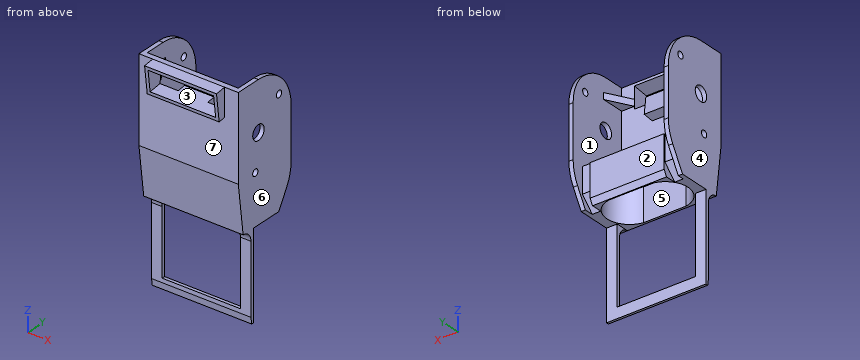
from build123d import *

# Parameters (mm, degrees)
EXTRUDE_1_DEPTH          = 15.5
SKETCH_2_W               = 41
SKETCH_2_H               = 24
EXTRUDE_2_DEPTH          = 2.5
EXTRUDE_3_DEPTH          = 41
EXTRUDE_5_DEPTH          = 1
EXTRUDE_6_DEPTH          = 1
EXTRUDE_7_DEPTH          = 2
CUT_EXTRUDE_1_REACH      = 81.452
SKETCH_10_R              = 1.6
SKETCH_10_R_2            = 3.5
EXTRUDE_8_DEPTH          = 2
CUT_EXTRUDE_2_REACH      = 82.601
SKETCH_12_R              = 3.5
SKETCH_12_R_2            = 1.6
EXTRUDE_9_DEPTH          = 43
EXTRUDE_10_DEPTH         = 3
EXTRUDE_11_DEPTH         = 1.5
FILLET_1_R               = 5
SKETCH_21_W              = 35
SKETCH_21_H              = 18
EXTRUDE_12_DEPTH         = 0.5
CHAMFER_1_SIZE           = 6
CUT_EXTRUDE_4_DEPTH      = 10
CUT_EXTRUDE_4_DEPTH_BACK = 0.7
SKETCH_24_W              = 99.76929375
SKETCH_24_H              = 144.1272379
CHAMFER_2_SIZE           = 15
CHAMFER_2_SIZE2          = 8.660254038
CHAMFER_3_SIZE           = 7.5
CHAMFER_3_SIZE2          = 12.990381057
CHAMFER_4_SIZE           = 1.5
CHAMFER_4_SIZE2          = 2.598076211
EXTRUDE_13_REACH         = 76.53
SKETCH_25_W              = 34
SKETCH_25_H              = 13
CUT_EXTRUDE_5_REACH      = 76.53
SKETCH_26_W              = 31
SKETCH_26_H              = 10
EXTRUDE_14_REACH         = 72.111
SKETCH_27_W              = 14
SKETCH_27_H              = 8
FILLET_2_R               = 20
FILLET_3_R               = 20


with BuildPart() as part:
    # ｽｹｯﾁ1 → ﾎﾞｽ - 押し出し1 (new body)
    with BuildSketch(Plane.XY):
        Polygon((10.055611053, 12.166632755), (-10.143634653, 12.166632755), (-20.595217471, 12.166632755), (-20.595217471, -0.083367245), (-20.595217471, -11.833367245), (-10.143634653, -11.833367245), (10.055611053, -11.833367245), (20.404782529, -11.833367245), (20.404782529, 0.125988678), (20.404782529, 12.166632755), align=None)
        with BuildLine():
            Line((9.95247038, 10.766632755), (-10.04752962, 10.766632755))
            ThreePointArc((-10.04752962, 10.766632755), (-19.245217471, 0.166632755), (-10.04752962, -10.433367245))
            Line((-10.04752962, -10.433367245), (9.95247038, -10.433367245))
            ThreePointArc((9.95247038, -10.433367245), (19.054782529, 0.166632755), (9.95247038, 10.766632755))
        make_face(mode=Mode.SUBTRACT)
    extrude(amount=EXTRUDE_1_DEPTH)

    # ｽｹｯﾁ2 → ﾎﾞｽ - 押し出し2 (add)
    with BuildSketch(Plane.XY.offset(15.5)):
        with Locations((-0.095217471, 0.166632755)):
            Rectangle(SKETCH_2_W, SKETCH_2_H)
    extrude(amount=EXTRUDE_2_DEPTH)

    # ｽｹｯﾁ3 → ﾎﾞｽ - 押し出し3 (add)
    with BuildSketch(Plane.ZY.offset(20.595217471)):
        Polygon((0, -12.15110343), (17.677739562, -14.384321281), (18, -11.833367245), (0, -11.833367245), align=None)
    extrude(amount=-EXTRUDE_3_DEPTH)

    # ｽｹｯﾁ5 → ﾎﾞｽ - 押し出し5 (add)
    with BuildSketch(Plane.ZY.offset(20.595217471)):
        Polygon((0, 12.166632755), (0, -12.15110343), (17.677739562, -14.384321281), (18, -11.833367245), (18, 12.166632755), align=None)
    extrude(amount=EXTRUDE_5_DEPTH)

    # ｽｹｯﾁ7 → ﾎﾞｽ - 押し出し6 (add)
    with BuildSketch(Plane(origin=(20.404782529, 0, 0), x_dir=(0, 0, -1), z_dir=(1, 0, 0))):
        Polygon((0, -12.15110343), (0, 12.166632755), (-18, 12.166632755), (-18, -11.833367245), (-17.677739562, -14.384321281), align=None)
    extrude(amount=EXTRUDE_6_DEPTH)

    # ｽｹｯﾁ8 → ﾎﾞｽ - 押し出し7 (add)
    with BuildSketch(Plane.ZY.offset(21.595217471)):
        Polygon((63, 0.066632755), (63, -14.384321281), (17.677739562, -14.384321281), (0, -12.15110343), (0, 12.166632755), (0, 17.84889657), (48, 17.84889657), (63, 17.84889657), align=None)
    extrude(amount=EXTRUDE_7_DEPTH)

    # ｽｹｯﾁ10 → ｶｯﾄ - 押し出し1 (cut, up to next)
    with BuildSketch(Plane.ZY.offset(23.595217471), mode=Mode.PRIVATE) as cut_extrude_1_sk1:
        with Locations((23.490675042, -4.00656608)):
            Circle(SKETCH_10_R)
    cut_extrude_1_tool1 = extrude(cut_extrude_1_sk1.sketch, amount=-CUT_EXTRUDE_1_REACH, mode=Mode.PRIVATE) & part.part
    # ｽｹｯﾁ10 → ｶｯﾄ - 押し出し1 (cut, up to next)
    with BuildSketch(Plane.ZY.offset(23.595217471), mode=Mode.PRIVATE) as cut_extrude_1_sk2:
        with Locations((50.912685274, 10.451419771)):
            Circle(SKETCH_10_R)
    cut_extrude_1_tool2 = extrude(cut_extrude_1_sk2.sketch, amount=-CUT_EXTRUDE_1_REACH, mode=Mode.PRIVATE) & part.part
    # ｽｹｯﾁ10 → ｶｯﾄ - 押し出し1 (cut, up to next)
    with BuildSketch(Plane.ZY.offset(23.595217471), mode=Mode.PRIVATE) as cut_extrude_1_sk3:
        with Locations((40, -2.085059006)):
            Circle(SKETCH_10_R_2)
    cut_extrude_1_tool3 = extrude(cut_extrude_1_sk3.sketch, amount=-CUT_EXTRUDE_1_REACH, mode=Mode.PRIVATE) & part.part
    add(cut_extrude_1_tool1.solids().sort_by_distance((-23.595217, -4.006566, 23.490675))[0], mode=Mode.SUBTRACT)
    add(cut_extrude_1_tool2.solids().sort_by_distance((-23.595217, 10.45142, 50.912685))[0], mode=Mode.SUBTRACT)
    add(cut_extrude_1_tool3.solids().sort_by_distance((-23.595217, -2.085059, 40))[0], mode=Mode.SUBTRACT)

    # ｽｹｯﾁ11 → ﾎﾞｽ - 押し出し8 (add)
    with BuildSketch(Plane(origin=(21.404782529, 0, 0), x_dir=(0, 0, -1), z_dir=(1, 0, 0))):
        Polygon((-63, -14.384321281), (-17.677739562, -14.384321281), (0, -12.15110343), (0, 17.84889657), (-63, 17.84889657), align=None)
    extrude(amount=EXTRUDE_8_DEPTH)

    # ｽｹｯﾁ12 → ｶｯﾄ - 押し出し2 (cut, up to next)
    with BuildSketch(Plane(origin=(23.404782529, 0, 0), x_dir=(0, 0, -1), z_dir=(1, 0, 0)), mode=Mode.PRIVATE) as cut_extrude_2_sk1:
        with Locations(Location((-40, -2.085059006, 0), (0, 0, 180))):
            Circle(SKETCH_12_R)
    cut_extrude_2_tool1 = extrude(cut_extrude_2_sk1.sketch, amount=-CUT_EXTRUDE_2_REACH, mode=Mode.PRIVATE) & part.part
    # ｽｹｯﾁ12 → ｶｯﾄ - 押し出し2 (cut, up to next)
    with BuildSketch(Plane(origin=(23.404782529, 0, 0), x_dir=(0, 0, -1), z_dir=(1, 0, 0)), mode=Mode.PRIVATE) as cut_extrude_2_sk2:
        with Locations(Location((-50.912685274, 10.451419771, 0), (0, 0, 180))):
            Circle(SKETCH_12_R_2)
    cut_extrude_2_tool2 = extrude(cut_extrude_2_sk2.sketch, amount=-CUT_EXTRUDE_2_REACH, mode=Mode.PRIVATE) & part.part
    # ｽｹｯﾁ12 → ｶｯﾄ - 押し出し2 (cut, up to next)
    with BuildSketch(Plane(origin=(23.404782529, 0, 0), x_dir=(0, 0, -1), z_dir=(1, 0, 0)), mode=Mode.PRIVATE) as cut_extrude_2_sk3:
        with Locations(Location((-23.490675042, -4.00656608, 0), (0, 0, 180))):
            Circle(SKETCH_12_R_2)
    cut_extrude_2_tool3 = extrude(cut_extrude_2_sk3.sketch, amount=-CUT_EXTRUDE_2_REACH, mode=Mode.PRIVATE) & part.part
    add(cut_extrude_2_tool1.solids().sort_by_distance((23.404783, -2.085059, 40))[0], mode=Mode.SUBTRACT)
    add(cut_extrude_2_tool2.solids().sort_by_distance((23.404783, 10.45142, 50.912685))[0], mode=Mode.SUBTRACT)
    add(cut_extrude_2_tool3.solids().sort_by_distance((23.404783, -4.006566, 23.490675))[0], mode=Mode.SUBTRACT)

    # ｽｹｯﾁ13 → ﾎﾞｽ - 押し出し9 (add)
    with BuildSketch(Plane.ZY.offset(-21.404782529)):
        Polygon((17.677739562, -14.384321281), (18, -11.833367245), (63, -11.833367245), (63, -14.384321281), align=None)
    extrude(amount=EXTRUDE_9_DEPTH)

    # ｽｹｯﾁ18 → ﾎﾞｽ - 押し出し10 (add)
    with BuildSketch(Plane.XY.offset(56)):
        Polygon((21.404782529, -0.833367245), (15.404782529, -11.833367245), (21.404782529, -11.833367245), align=None)
    extrude_10 = extrude(amount=-EXTRUDE_10_DEPTH)

    # ﾐﾗｰ2: ﾎﾞｽ - 押し出し10 across plane
    add(extrude_10.mirror(Plane(origin=(0, 0, 0), x_dir=(0, 0, 1), z_dir=(1, 0, 0))))

    # ｽｹｯﾁ20 → ﾎﾞｽ - 押し出し11 (add)
    with BuildSketch(Plane(origin=(0, -5.15110343, 0), x_dir=(1, 0, 0), z_dir=(0, 1, 0))):
        Polygon((23.404782529, 0), (18.404782529, 0), (18.404782529, 5), (18.404782529, 36), (-18.595217471, 36), (-18.595217471, 5), (-18.595217471, 0), (-23.595217471, 0), (-23.595217471, 41), (23.404782529, 41), align=None)
    extrude(amount=-EXTRUDE_11_DEPTH)

    # ﾌｨﾚｯﾄ1
    fillet_1_edges = [part.edges().sort_by_distance(p)[0] for p in [
        (20.904782529, -6.65110343, 0),
        (-21.095217471, -6.65110343, 0),
    ]]
    fillet(fillet_1_edges, radius=FILLET_1_R)

    # ｽｹｯﾁ21 → ﾎﾞｽ - 押し出し12 (add)
    with BuildSketch(Plane(origin=(0, 12.166632755, 0), x_dir=(1, 0, 0), z_dir=(0, 1, 0))):
        with Locations((-0.095217471, -9)):
            Rectangle(SKETCH_21_W, SKETCH_21_H)
    extrude(amount=EXTRUDE_12_DEPTH)

    # 面取り1
    chamfer_1_edges = [part.edges().sort_by_distance(p)[0] for p in [
        (19.404782529, 12.166632755, 0),
        (-19.595217471, 12.166632755, 0),
    ]]
    chamfer(chamfer_1_edges, length=CHAMFER_1_SIZE)

    # ｽｹｯﾁ24 → ｶｯﾄ - 押し出し4 (cut, two sides: drawn at the far end of the back side and taken through both)
    with BuildSketch(Plane(origin=(0, -11.960228801, -1.51092827), x_dir=(1, 0, 0), z_dir=(0, -0.9921147013144787, -0.12533323356429749)).offset(-CUT_EXTRUDE_4_DEPTH_BACK)):
        with Locations((0, 9.634165713)):
            Rectangle(SKETCH_24_W, SKETCH_24_H)
    extrude(amount=CUT_EXTRUDE_4_DEPTH + CUT_EXTRUDE_4_DEPTH_BACK, mode=Mode.SUBTRACT)

    # 面取り2
    chamfer_2_edges = [part.edges().sort_by_distance(p)[0] for p in [
        (-22.595217471, 17.84889657, 0),
    ]]
    chamfer_2_side = [part.faces().sort_by_distance(p)[0] for p in [
        (-22.595217471, 17.84889657, 31.5),
    ]]
    chamfer(chamfer_2_edges, length=CHAMFER_2_SIZE, length2=CHAMFER_2_SIZE2, reference=chamfer_2_side[0])

    # 面取り3
    chamfer_3_edges = [part.edges().sort_by_distance(p)[0] for p in [
        (22.404782529, 17.84889657, 0),
    ]]
    chamfer_3_side = [part.faces().sort_by_distance(p)[0] for p in [
        (-23.041397644, 2.018769551, 0),
    ]]
    chamfer(chamfer_3_edges, length=CHAMFER_3_SIZE, length2=CHAMFER_3_SIZE2, reference=chamfer_3_side[0])

    # 面取り4
    chamfer_4_edges = [part.edges().sort_by_distance(p)[0] for p in [
        (-0.095217471, 12.666632755, 0),
    ]]
    chamfer_4_side = [part.faces().sort_by_distance(p)[0] for p in [
        (22.876540457, 2.59889657, 0),
    ]]
    chamfer(chamfer_4_edges, length=CHAMFER_4_SIZE, length2=CHAMFER_4_SIZE2, reference=chamfer_4_side[0])

    # ｽｹｯﾁ25 → ﾎﾞｽ - 押し出し13 (add, up to next)
    with BuildSketch(Plane(origin=(0, -11.26574851, -1.423195007), x_dir=(1, 0, 0), z_dir=(0, -0.9921147013144788, -0.12533323356429746)), mode=Mode.PRIVATE) as extrude_13_sk1:
        with Locations((-0.095217471, 57.806059682)):
            Rectangle(SKETCH_25_W, SKETCH_25_H)
    extrude_13_tool1 = extrude(extrude_13_sk1.sketch, amount=-EXTRUDE_13_REACH, mode=Mode.PRIVATE) - part.part
    add(extrude_13_tool1.solids().sort_by_distance((-0.095217, -18.510769, 55.927047))[0])

    # ｽｹｯﾁ26 → ｶｯﾄ - 押し出し5 (cut, up to next)
    with BuildSketch(Plane(origin=(0, -11.26574851, -1.423195007), x_dir=(1, 0, 0), z_dir=(0, -0.9921147013144788, -0.1253332335642974)), mode=Mode.PRIVATE) as cut_extrude_5_sk1:
        with Locations((-0.095217471, 57.806059682)):
            Rectangle(SKETCH_26_W, SKETCH_26_H)
    cut_extrude_5_tool1 = extrude(cut_extrude_5_sk1.sketch, amount=-CUT_EXTRUDE_5_REACH, mode=Mode.PRIVATE) & part.part
    add(cut_extrude_5_tool1.solids().sort_by_distance((-0.095217, -18.510769, 55.927047))[0], mode=Mode.SUBTRACT)

    # ﾎﾞｽ - 押し出し14: up to this plane
    extrude_14_end = Plane(origin=(-66.989211101, -11.833367245, 18), z_dir=(0, -1, 0))
    # ｽｹｯﾁ27 → ﾎﾞｽ - 押し出し14 (add, up to the surface)
    with BuildSketch(Plane(origin=(0, -1.344601497, -0.169862671), x_dir=(-1, 0, 0), z_dir=(0, -0.9921147013144788, -0.1253332335642974)), mode=Mode.PRIVATE) as extrude_14_sk1:
        with Locations((0, -48.806059682)):
            Rectangle(SKETCH_27_W, SKETCH_27_H)
    extrude_14_tool1 = split(extrude(extrude_14_sk1.sketch, amount=EXTRUDE_14_REACH, mode=Mode.PRIVATE), bisect_by=extrude_14_end, keep=Keep.BOTH, mode=Mode.PRIVATE)
    add(extrude_14_tool1.solids().sort_by_distance((0, -7.461623, 48.251347))[0])

    # ﾌｨﾚｯﾄ2
    fillet_2_edges = [part.edges().sort_by_distance(p)[0] for p in [
        (-22.595217471, 17.84889657, 63),
        (22.404782529, 17.84889657, 63),
    ]]
    fillet(fillet_2_edges, radius=FILLET_2_R)

    # ﾌｨﾚｯﾄ3
    fillet_3_edges = [part.edges().sort_by_distance(p)[0] for p in [
        (-22.595217471, 17.84889657, 15),
        (22.404782529, 17.84889657, 12.990381057),
    ]]
    fillet(fillet_3_edges, radius=FILLET_3_R)


solid = part.part
Read the model definition and answer for the solid it produces. Units are mm, in the model's axes. Face numbers are marked on the shaded views. A direction names the side the tool comes from. Coordinates: 2 decimals unless noted, no trailing zeros. Order: outer loops, then holes, each group sorted by start corner. A loop starts at its lowest first (then second) coordinate and runs counter-clockwise, first axis right, second up. Notation, with made-up numbers: M -4.5,2 L 53.5,2 A15 ccw 53.5,17 Z; hole C 12.25,65 d10. An arc over 180 degrees is marked long. Put each result on its own line as item: value. Start each with the question number.
Item 1: Consider probe 1 along X at (y, z) = (1.5, 45); probe 2 along Y at (x, z) = (-22.1, 40); probe 3 along Z at (x, y) = (7, -0.5). Determine where each line is inside the solid, lowest interval first. Write a range as [from, to].
Item 2: Given pin 1 Ø6 at (y, z) = (-16, 56.5) entering from +X; pin 2 Ø8 at (x, z) = (-15.5, -29) entering from +Y; pin 3 Ø10 at (x, z) = (-0.5, 39.5) entering from -Y; pin 4 Ø2.5 at (y, z) = (-17.5, 59.5) entering from -X, each flat-ended and moving along its own axis, determine where each tip first touches the part or whether it passes through.
Item 3: Section D-D, the plane z = -1.5 is taken. Determine the outline of the cut face in (x, y).
Item 4: Section C-C, the plane z = 40 is taken. Determine the outline of the cut face in (x, y).
Item 5: The mould has two halves that part along X. Classify the marked faces 4, 5, 6 and 7: +X half, -X half, draft (parallel to the pull), parting line (faces both ways), or undercut.
Item 6: For the marked faces 1, 2 and 3, determine the directions among +Z, -Z, +X, -X, +Y, -Y from which every point of the face is accessible in a straight line to the end or side of a thin tool.
Item 7: Section B-B, the plane z = -30 is taken. Determine the outline of the cut face in (x, y).
Item 8: Section A-A, the plane x = -5.5 is taken. Determine the outline of the cut face in (y, z).
Computed:
1. probe 1: x = [-23.6, -21.6], [21.4, 23.4]
1. probe 2: y = [-14.38, -5.59], [1.41, 17.85]
1. probe 3: z = [15.5, 18]
2. pin 1: stops at x = 23.4
2. pin 2: stops at y = -5.15
2. pin 3: stops at y = -14.38
2. pin 4: stops at x = -17.1
3. outline: M -23.6,-8.08 L -18.6,-8.08 L -18.6,-5.15 L -23.6,-5.15 Z; M 18.4,-8.08 L 23.4,-8.08 L 23.4,-5.15 L 18.4,-5.15 Z
4. outline: M -23.6,-14.38 L 23.4,-14.38 L 23.4,-5.59 L 21.4,-5.59 L 21.4,-11.83 L -21.6,-11.83 L -21.6,-5.59 L -23.6,-5.59 Z; M -23.6,1.41 L -21.6,1.41 L -21.6,17.85 L -23.6,17.85 Z; M 21.4,1.41 L 23.4,1.41 L 23.4,17.85 L 21.4,17.85 Z
5. face 4: -X half
5. face 5: undercut
5. face 6: +X half
5. face 7: draft
6. face 1: +Y
6. face 2: +Z, -Z, +Y
6. face 3: -Y
7. outline: M -23.6,-6.65 L -18.6,-6.65 L -18.6,-5.15 L -23.6,-5.15 Z; M 18.4,-6.65 L 23.4,-6.65 L 23.4,-5.15 L 18.4,-5.15 Z
8. outline: M -19.33,62.38 L -19.14,60.89 L -11.83,61.81 L -11.83,63 L -14.38,63 Z; M -17.88,50.97 L -17.7,49.48 L -14.38,49.9 L -14.38,23.26 L -11.45,0 L -10.43,0 L -10.43,15.5 L 10.77,15.5 L 10.77,0 L 11.17,0 L 12.67,2.6 L 12.67,18 L -11.83,18 L -11.83,43.67 L -6.96,44.28 L -7.96,52.22 Z; M -6.65,-37.95 L -6.27,-41 L -5.15,-41 L -5.15,-36 L -6.65,-36 Z
